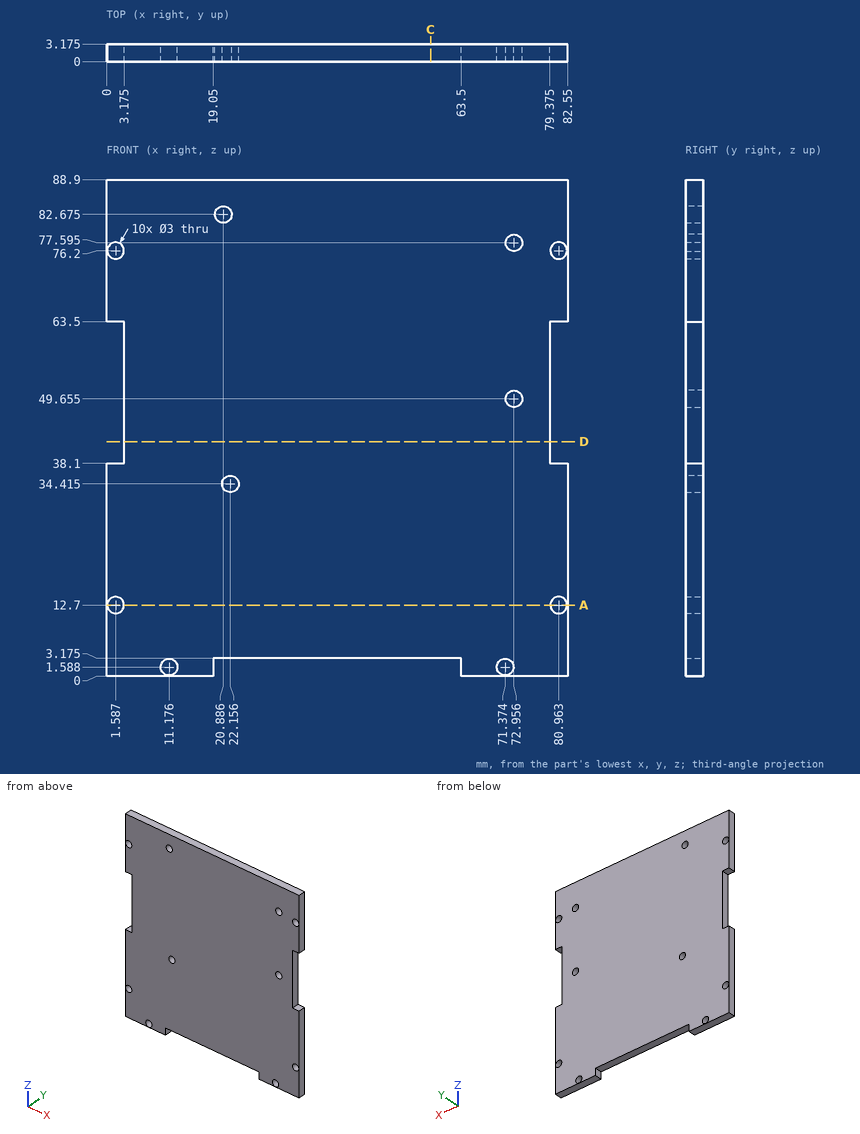
Geometry check sheet. Reference: drawing and pictorial views, mm from the part's lowest x, y, z. Give positions to 0.01 mm unless a question says otherwise; leave off trailing zeros. Loops run counter-clockwise (first coordinate to the right, second up) from the corner with the lowest first, then second, coordinate; pieces in that order, holes last.
1. Section check D-D, the plane z = 42. Enter the section's corners in (x, y) (1 decimal).
2. Go/stop test with flat-tipped pins: pin 1 Ø1.6 at (y, z) = (2, 49.5) entering from -X (1 decimal); pin 2 Ø1 at (x, y) = (50.5, 1) entering from -Z (1 decimal); pin 3 Ø1.6 at (y, z) = (1, 46.5) entering from +X (1 decimal). Record where each tip stops, or that it passes through.
3. Thickness scan on line 1 (Z direction, x = 32, y = 1.9) (1 decimal); line 2 (X direction, y = 2.8, z = 78); line 3 (X direction, y = 0.5, z = 46.5) (1 decimal). Record the ranges inside material, lowest first.
4. Section check A-A, the plane z = 12.7. Count the separate pieces of the cut face and the enclosed holes in it, then the cut area to 3 significant figures.
5. Section check C-C, the plane x = 58. Enter the section's corners in (y, z) (1 decimal), then the cut area to 3 significant figures.
Geometry says:
1. outline: (3.2, 0) - (79.4, 0) - (79.4, 3.2) - (3.2, 3.2) - close
2. pin 1: stops at x = 3.2
2. pin 2: stops at z = 3.2
2. pin 3: stops at x = 79.4
3. line 1: z = 3.2 to 88.9
3. line 2: x = 0 to 71.51, 74.4 to 82.55
3. line 3: x = 3.2 to 79.4
4. separate pieces: 3
4. enclosed holes: 0
4. area: 243 mm2
5. outline: (0, 3.2) - (3.2, 3.2) - (3.2, 88.9) - (0, 88.9) - close
5. area: 272 mm2
